Read the model definition and answer for the solid it produces. Units are mm, in the model's axes. Coordinates: 2 decimals unless noted, no trailing zeros. Order: outer loops, then holes, each group sorted by start corner. A loop starts at its lowest first (then second) coordinate and runs counter-clockwise, first axis right, second up. Notation, with made-up numbers: (81.5, 20.25) -> (125.5, 20.25) arc R6 cw to (125.5, 26.25) -> close; hole circle Ø11 at (15.25, -7). An arc over 180 degrees is marked (long way). Answer in a Markdown table with one row per item.
from build123d import *

# Parameters (mm, degrees)
SKETCH_W   = 95
SKETCH_H   = 70
SKETCH_R   = 8
SKETCH_R_2 = 9.5
PAD_DEPTH  = 10


with BuildPart() as part:
    # Sketch → Pad (new body)
    with BuildSketch(Plane.XY):
        with Locations((27.5, -15)):
            Rectangle(SKETCH_W, SKETCH_H)
        Circle(SKETCH_R, mode=Mode.SUBTRACT)
        with Locations((0, -30)):
            Circle(SKETCH_R_2, mode=Mode.SUBTRACT)
    extrude(amount=PAD_DEPTH)


solid = part.part
Q1. Consider line 1 (Y direction, x = 0, z = 8); line 2 (X direction, y = 0.5, z = 5.5); line 3 (Y direction, x = -1, z = 1). Determine where each line is inside the solid, lowest interval first.
Outcome:
| item | result |
|---|---|
| line 1 | -50 to -39.5, -20.5 to -8, 8 to 20 |
| line 2 | -20 to -7.98, 7.98 to 75 |
| line 3 | -50 to -39.45, -20.55 to -7.94, 7.94 to 20 |
Q2. The part is cut by section D-D (y = -30). Write down the section's boundary in (x, z), then the cut area to 3 significant figures.
Outcome:
| item | result |
|---|---|
| outline | (-20, 0) -> (-9.5, 0) -> (-9.5, 10) -> (-20, 10) -> close; (9.5, 0) -> (75, 0) -> (75, 10) -> (9.5, 10) -> close |
| area | 760 mm² |
Q3. Given pin 1 (6 mm diameter, centred on x = 45.5, y = -26, fed in from -Z); pin 2 (15 mm diameter, centred on x = 0, y = -30, fed in from -Z), each flat-ended and moving along its own axis, determine where each tip first touches the part or whether it passes through.
Outcome:
| item | result |
|---|---|
| pin 1 | z = 0 |
| pin 2 | through |
Q4. The part is cut by section C-C (z = 2.25). Write down the section's boundary in (x, y), then the cut area to 3 significant figures.
Outcome:
| item | result |
|---|---|
| outline | (-20, -50) -> (75, -50) -> (75, 20) -> (-20, 20) -> close; hole circle Ø19 at (0, -30); hole circle Ø16 at (0, 0) |
| area | 6,170 mm² |
Q5. For a pull along Y with two mould halves and no side action, classify faces 1 (the face through (27, -50, 5)), 2 (the face through (-1.73, -7.81, 4.93)), 3 (the face through (27, -15, 0)) as pulls with the +Y half, pulls with the -Y half, needs draft (parallel to the pull), parting line crosses it, or undercut.
Outcome:
| item | result |
|---|---|
| face 1 | pulls with the -Y half |
| face 2 | undercut |
| face 3 | needs draft |
Q6. The part is cut by section A-A (y = 0). Write down the section's boundary in (x, z).
Outcome:
| item | result |
|---|---|
| outline | (-20, 0) -> (-8, 0) -> (-8, 10) -> (-20, 10) -> close; (8, 0) -> (75, 0) -> (75, 10) -> (8, 10) -> close |
Q7. The part is cut by section B-B (x = 0). Write down the section's boundary in (y, z), then the cut area to 3 significant figures.
Outcome:
| item | result |
|---|---|
| outline | (-50, 0) -> (-39.5, 0) -> (-39.5, 10) -> (-50, 10) -> close; (-20.5, 0) -> (-8, 0) -> (-8, 10) -> (-20.5, 10) -> close; (8, 0) -> (20, 0) -> (20, 10) -> (8, 10) -> close |
| area | 350 mm² |
